Read the model definition and answer for the solid it produces. Units are mm, in the model's axes. A direction names the side the tool comes from. Give positions to 0.01 mm unless a question says otherwise; leave off trailing zeros. Order: outer loops, then holes, each group sorted by start corner. A loop starts at its lowest first (then second) coordinate and runs counter-clockwise, first axis right, second up. Notation, with made-up numbers: M 30.25,-31.5 L 76.25,-31.5 A25 cw 76.25,-5.5 Z; hole C 27,-17 d4. An arc over 180 degrees is marked long. One line per item, written item: value.
from build123d import *

# Parameters (mm, degrees)
SZKIC2_W                    = 10
SZKIC2_H                    = 13
DODANIE_WYCI_GNI_CIE1_DEPTH = 6
SZKIC4_W                    = 24
SZKIC4_H                    = 9.5


with BuildPart() as part:
    # Szkic1 → Obrót1 (revolve)
    with BuildSketch(Plane.XY, mode=Mode.PRIVATE) as obr_t1_sk:
        Polygon((0, 0), (0, 11.08), (0.92, 12), (12, 12), (12, 0), align=None)
    revolve(obr_t1_sk.sketch.rotate(Axis((12, 0, 0), (-1, 0, 0)), 270), axis=Axis((12, 0, 0), (-1, 0, 0)))

    # Szkic2 → Obrót2 (revolve)
    with BuildSketch(Plane.XY, mode=Mode.PRIVATE) as obr_t2_sk:
        with Locations((17, 6.5)):
            Rectangle(SZKIC2_W, SZKIC2_H)
    revolve(obr_t2_sk.sketch.rotate(Axis((22, 0, 0), (-1, 0, 0)), 270), axis=Axis((22, 0, 0), (-1, 0, 0)))

    # Szkic3 → Dodanie-wyciągnięcie1 (add)
    with BuildSketch(Plane(origin=(22, 0, 0), x_dir=(0, 0, -1), z_dir=(1, 0, 0))):
        Polygon((-13.5, 7.794228634), (-13.5, -7.794228634), (0, -15.588457268), (13.5, -7.794228634), (13.5, 7.794228634), (0, 15.588457268), align=None)
    extrude(amount=DODANIE_WYCI_GNI_CIE1_DEPTH)

    # Szkic4 → Obrót3 (revolve)
    with BuildSketch(Plane.XY, mode=Mode.PRIVATE) as obr_t3_sk:
        with Locations((40, 4.75)):
            Rectangle(SZKIC4_W, SZKIC4_H)
    revolve(obr_t3_sk.sketch.rotate(Axis((52, 0, 0), (-1, 0, 0)), 270), axis=Axis((52, 0, 0), (-1, 0, 0)))

    # Szkic5 → Obrót4 (revolve)
    with BuildSketch(Plane.XY, mode=Mode.PRIVATE) as obr_t4_sk:
        with BuildLine():
            Line((52, 0), (52, 10))
            Line((52, 10), (57, 9.5))
            Line((57, 9.5), (57, 10))
            Line((57, 10), (61.597042092, 9.090492439))
            ThreePointArc((61.597042092, 9.090492439), (61.886342494, 8.917394828), (62, 8.6))
            Line((62, 8.6), (62, 0))
            Line((62, 0), (52, 0))
        make_face()
    revolve(obr_t4_sk.sketch.rotate(Axis((62, 0, 0), (-1, 0, 0)), 270), axis=Axis((62, 0, 0), (-1, 0, 0)))

    # Szkic6 → Wycięcie-obrót1 (revolve, cut)
    with BuildSketch(Plane.XY, mode=Mode.PRIVATE) as wyci_cie_obr_t1_sk:
        Polygon((0, 0), (0, 7.207106781), (0.707106781, 6.5), (62, 6.5), (62, 0), align=None)
    revolve(wyci_cie_obr_t1_sk.sketch.rotate(Axis((62, 0, 0), (-1, 0, 0)), 270), axis=Axis((62, 0, 0), (-1, 0, 0)), mode=Mode.SUBTRACT)

    # Szkic7 → Wycięcie-obrót2 (revolve, cut)
    with BuildSketch(Plane.XY):
        Polygon((22, 13.5), (29.794228634, 27), (22, 27), align=None)
    revolve(axis=Axis((22, 0, 0), (-1, 0, 0)), mode=Mode.SUBTRACT)

    # Szkic8 → Wycięcie-obrót3 (revolve, cut)
    with BuildSketch(Plane.XY):
        Polygon((20.205771366, 27), (28, 13.5), (28, 27), align=None)
    revolve(axis=Axis((22, 0, 0), (-1, 0, 0)), mode=Mode.SUBTRACT)


solid = part.part
1) Find section A-A, the plane x = 47. Write down the section's boundary in (y, z), plus the area to 3 significant figures.
Reported:
outline: C 0,0 d19; hole C 0,0 d13
area: 151 mm^2
2) Each of these flat-tipped pins is pushed along its axis until it touches: pin 1 Ø6 at (x, z) = (37, -4) entering from -Y; pin 2 Ø1.5 at (x, y) = (13, 10) entering from -Z; pin 3 Ø10 at (x, y) = (38.5, -3.5) entering from -Z. Where does it stop, or does it pass through?
Reported:
pin 1: stops at y = -9.45
pin 2: stops at z = -9.13
pin 3: stops at z = -9.5
3) Which of the six approach directions +Z, -Z, +X, -X, +Y, -Y give full straight-line access (tool end or side, diameter ignored) to faces 1 (the face through (61.37, -8.92, -1.98)), 2 (the face through (22, 11.1, 7.1)), 3 (the face through (55.65, 2.89, 9.19))?
Reported:
face 1: +X
face 2: -X
face 3: none
4) Consider probe 1 along Y at (x, z) = (46, 0); probe 2 along Y at (x, z) = (24, 0); probe 3 along X at (y, z) = (13, -1.5). Determine where each line is inside the solid, lowest interval first.
Reported:
probe 1: y = -9.5 to -6.5, 6.5 to 9.5
probe 2: y = -15.59 to -6.5, 6.5 to 15.59
probe 3: x = 22 to 28
